from build123d import *

# Parameters (mm, degrees)
ESQUISSE1_W                  = 20
ESQUISSE1_H                  = 60
BOSS_EXTRU_1_DEPTH           = 10
ENL_V_MAT_EXTRU_1_DEPTH      = 65.031242374
ENL_V_MAT_EXTRU_1_DEPTH_BACK = 65.031242374
ESQUISSE2_R                  = 5
ESQUISSE2_R_2                = 2.5
CONG_1_R                     = 10


with BuildPart() as part:
    # Esquisse1 → Boss.-Extru.1 (new body)
    with BuildSketch(Plane.XY):
        with Locations((10, 30)):
            Rectangle(ESQUISSE1_W, ESQUISSE1_H)
    extrude(amount=BOSS_EXTRU_1_DEPTH)

    # Esquisse2 → Enlèv. mat.-Extru.1 (cut, two sides: drawn at the far end of the back side and taken through both)
    with BuildSketch(Plane.XY.offset(10).offset(-ENL_V_MAT_EXTRU_1_DEPTH_BACK)):
        with Locations((10, 50)):
            Circle(ESQUISSE2_R)
        with Locations((10, 10)):
            Circle(ESQUISSE2_R_2)
    extrude(amount=ENL_V_MAT_EXTRU_1_DEPTH + ENL_V_MAT_EXTRU_1_DEPTH_BACK, mode=Mode.SUBTRACT)

    # Congé1
    cong_1_edges = [part.edges().sort_by_distance(p)[0] for p in [
        (0, 0, 5),
        (20, 0, 5),
        (0, 60, 5),
        (20, 60, 5),
    ]]
    fillet(cong_1_edges, radius=CONG_1_R - 0.0001)  # a hair under: the kernel refuses the full size


solid = part.part
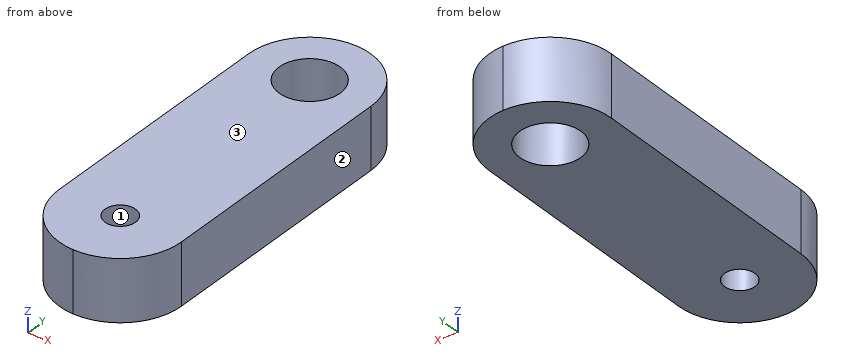
Work out the finished part from the listing and answer in its coordinate system (mm). Face numbers are marked on the shaded views. Coordinates: 2 decimals unless noted, no trailing zeros. Write each loop counter-clockwise with the first axis right and the second up, starting at its lowest first coordinate (ties: lowest second). Pieces come first, ordered by that corner, then holes. Notation, with made-up numbers: (-40, 33) - (-4, 33) arc R22 ccw to (-4, 60) - close; hole circle Ø5 at (-29, -13). An arc over 180 degrees is marked (long way). One line per question, with ' | ' between items.
1) Find section B-B, the plane x = 17.25. Determine the outline of the cut face in (y, z), and give its area (3 significant figures).
Checks:
outline: (3.11, 0) - (56.89, 0) - (56.89, 10) - (3.11, 10) - close | area: 538 mm2
2) Consider probe 1 along Y at (x, z) = (10, 4.5); probe 2 along X at (y, z) = (50, 8.25); probe 3 along Y at (x, z) = (11.5, 9.25). Determine where each line is inside the solid, lowest interval first. Write a range as [from, to].
Checks:
probe 1: [0, 7.5], [12.5, 45], [55, 60] | probe 2: [0, 5], [15, 20] | probe 3: [0.11, 8], [12, 45.23], [54.77, 59.89]
3) The mould has two halves that part along X. Classify the marked faces 1, 2 and 3: +X half, -X half, draft (parallel to the pull), parting line (faces both ways), or undercut.
Checks:
face 1: undercut | face 2: +X half | face 3: draft
4) Find section A-A, the plane z = 5. Give the number of separate pieces and of enclosed holes in the cut face, and give its area (3 significant figures).
Checks:
separate pieces: 1 | enclosed holes: 2 | area: 1,020 mm2
5) Flat-ended cylindrical pins translate along their axes: P1, Ø5, axis at x = 15, z = 2, coming from the -Y side; P2, Ø1, axis at x = 17.5, z = 1.5, coming from the -Y side. Find the tip coordinate at first contact, or state that the pin passes through.
Checks:
P1: y = 0.32 | P2: y = 2.86
